Autodesk Inventor part; units mm, degrees
ref_plane "YZ Plane" through (0, 0, 0) normal (1, 0, 0) x (0, 1, 0)
ref_plane "XZ Plane" through (0, 0, 0) normal (0, 1, 0) x (-1, 0, 0)
ref_plane "XY Plane" through (0, 0, 0) normal (0, 0, 1) x (1, 0, 0)
sketch "Sketch1" plane through (0, 0, 0) normal (0, 0, 1) x (1, 0, 0)
  line L0 (-12.7, -12.7) -> (12.7, -12.7)
  line L1 (12.7, -12.7) -> (12.7, 12.7)
  line L2 (12.7, 12.7) -> (-12.7, 12.7)
  line L3 (-12.7, 12.7) -> (-12.7, -12.7)
  line L4 (-12.7, -12.7) -> (12.7, 12.7) construction
  line L5 (12.7, -12.7) -> (-12.7, 12.7) construction
  line L6 (-9.525, -9.525) -> (9.525, -9.525)
  line L7 (9.525, -9.525) -> (9.525, 9.525)
  line L8 (9.525, 9.525) -> (-9.525, 9.525)
  line L9 (-9.525, 9.525) -> (-9.525, -9.525)
  line L10 (-9.525, -9.525) -> (9.525, 9.525) construction
  line L11 (9.525, -9.525) -> (-9.525, 9.525) construction
  point P0 (0, 0)
  dimension "d0" = 25.4
  dimension "d1" = 25.4
  dimension "d2" = 3.175
  dimension "d3" = 3.175
extrude "Extrusion1" add sketch "Sketch1" along normal mid plane 203.2
properties part number "8-inchAluminumTubing"
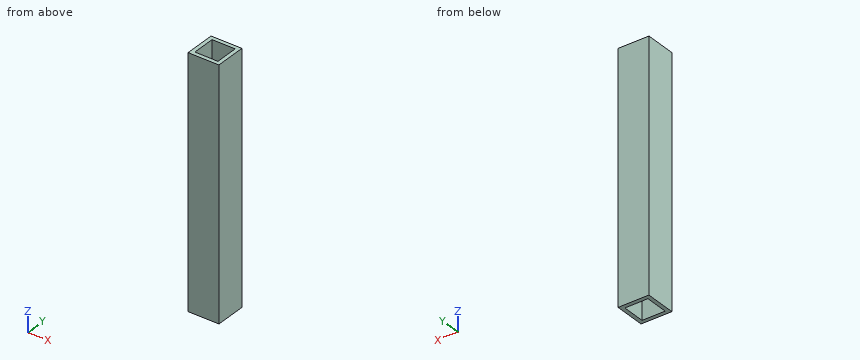
Model file for the job. Use its own axes, mm. Round coordinates to 2 decimals unless told otherwise and drop trailing zeros. Order: outer loops, then holes, each group sorted by start corner. A loop starts at its lowest first (then second) coordinate and runs counter-clockwise, first axis right, second up. Notation, with made-up numbers: M 78,28 L 130,28 A15 ccw 130,40 Z; hole C 58.5,-29 d8. An arc over 180 degrees is marked long. Write each question's results on one line, items separated by ' | '. Start each with the question number.
(1) Saw through at A-A, the plane y = 7. Give the cut face in (x, z) (3 decimals).
(2) Saw through at C-C, the plane z = 18.5. Give the cut face in (x, y) (3 decimals), then the cut area to 3 significant figures.
(3) Probe probe 1 along X at (y, z) = (4.5, 63.5) (3 decimals). List the from-to ranges inside material, lowest first. Write a range as from..to.
Established:
1) outline: M -12.7,-101.6 L -9.525,-101.6 L -9.525,101.6 L -12.7,101.6 Z; M 9.525,-101.6 L 12.7,-101.6 L 12.7,101.6 L 9.525,101.6 Z
2) outline: M -12.7,-12.7 L 12.7,-12.7 L 12.7,12.7 L -12.7,12.7 Z; hole M -9.525,-9.525 L 9.525,-9.525 L 9.525,9.525 L -9.525,9.525 Z | area: 282 mm^2
3) probe 1: x = -12.7..-9.525, 9.525..12.7
